Could you check a few things on this model? Use its own coordinates, in mm. Give positions to 0.01 mm unless a question says otherwise; leave off trailing zeros. Loops run counter-clockwise (first coordinate to the right, second up) from the corner with the lowest first, then second, coordinate; pieces in that order, holes last. Notation, with made-up numbers: (-31.75, 21.5) - (2.25, 21.5) arc R10 ccw to (2.25, 40.5) - close; hole circle Ø9 at (4.25, 44). An arc over 180 degrees is marked (long way). Write each question's results on one line, items separated by ' | '. Start each with the question number.
1) I want a section at D-D, the plane y = 2.15. Count the separate pieces of the cut face and the enclosed holes in it, and give its area (3 significant figures).
2) I'm going to push a flat-ended pin straight in: pin 1 (5 mm diameter, centred on x = 12.5, z = 2, fed in from +Y). Where does the tip first touch, or does it pass through?
3) I want a section at C-C, the plane z = -12. Write out the boundary of the cut face in (x, y), and give its area (3 significant figures).
4) If we mould it in two halves opening along X, with no side actions, what happens to faces 1 (the face through (10.464, 1.318, 3.575)), 2 (the face through (0, 1, 17)), 3 (the face through (-17, 1, 0)), 4 (the face through (14.15, 1.32, -13.99))? For each: +X half, -X half, draft (parallel to the pull), parting line (faces both ways), or undercut.
5) I want a section at B-B, the plane x = -5.5. Write out the boundary of the cut face in (y, z).
6) If I drill on probe 1 along X at (y, z) = (1.95, -6); probe 2 along X at (y, z) = (0.6, -1.5); probe 3 along Z at (x, y) = (-8, 2.25), over which ranges is the centre line in solid material (lowest first)? Write a range as [from, to].
7) I want a section at A-A, the plane x = -1. Write out the boundary of the cut face in (y, z), and give its area (3 significant figures).
from build123d import *

# Parameters (mm, degrees)
SKETCH1_W                        = 34
SKETCH1_H                        = 34
BASE_DEPTH                       = 2.6
BASE_FILLET_R                    = 10
INNER_CUT_DEPTH                  = 25.181811347
INNER_LEFT_PROFILE_DEPTH         = 2.6
SKETCH5_R                        = 1.5
RIVET_HOLE_DEPTH                 = 25.181811347
GROOVED_PARTIAL_CIRCLE_CUT_DEPTH = 25.181811347
ILP_F_R                          = 0.5
IC_F_R                           = 1
ILP_F_OF_MIRROR_INNER_FEATURES_R = 0.5
IC_F_OF_MIRROR_INNER_FEATURES_R  = 1


with BuildPart() as part:
    # Sketch1 → BASE (new body)
    with BuildSketch(Plane(origin=(0, 0, 0), x_dir=(1, 0, 0), z_dir=(0, 1, 0))):
        Rectangle(SKETCH1_W, SKETCH1_H)
    extrude(amount=BASE_DEPTH)

    # BASE FILLET
    base_fillet_edges = [part.edges().sort_by_distance(p)[0] for p in [
        (17, 1.3, 17),
        (-17, 1.3, 17),
        (-17, 1.3, -17),
        (17, 1.3, -17),
    ]]
    fillet(base_fillet_edges, radius=BASE_FILLET_R)

    # Sketch3 → INNER CUT (cut, through all)
    with BuildSketch(Plane(origin=(0, 2.6, 0), x_dir=(1, 0, 0), z_dir=(0, 1, 0))):
        with BuildLine():
            Line((-10, -9.5), (10, -9.5))
            ThreePointArc((10, -9.5), (12.828427125, -8.328427125), (14, -5.5))
            Line((14, -5.5), (14, 7))
            ThreePointArc((14, 7), (11.949747468, 11.949747468), (7, 14))
            Line((7, 14), (-7, 14))
            ThreePointArc((-7, 14), (-11.949747468, 11.949747468), (-14, 7))
            Line((-14, 7), (-14, -5.5))
            ThreePointArc((-14, -5.5), (-12.828427125, -8.328427125), (-10, -9.5))
        make_face()
    extrude(amount=-INNER_CUT_DEPTH, mode=Mode.SUBTRACT)

    # Sketch4 → INNER LEFT PROFILE (add)
    with BuildSketch(Plane(origin=(0, 0, 0), x_dir=(1, 0, 0), z_dir=(0, 1, 0))):
        with BuildLine():
            Line((-4, 2.6), (-4, -9.5))
            Line((-4, -9.5), (0, -9.5))
            Line((0, -9.5), (0, 11))
            Line((0, 11), (-7, 11))
            ThreePointArc((-7, 11), (-9.828427125, 9.828427125), (-11, 7))
            Line((-11, 7), (-11, 0.6))
            ThreePointArc((-11, 0.6), (-11.5, -2.9), (-11, -6.4))
            Line((-11, -6.4), (-7, -6.4))
            ThreePointArc((-7, -6.4), (-6.5, -2.9), (-7, 0.6))
            Line((-7, 0.6), (-7, 2.6))
            ThreePointArc((-7, 2.6), (-5.5, 4.1), (-4, 2.6))
        make_face()
    inner_left_profile = extrude(amount=INNER_LEFT_PROFILE_DEPTH)

    # Sketch5 → RIVET HOLE (cut, through all)
    with BuildSketch(Plane(origin=(0, 2.6, 0), x_dir=(1, 0, 0), z_dir=(0, 1, 0))):
        with Locations(Location((-9, -3.9, 0), (0, 0, 270))):
            Circle(SKETCH5_R)
    rivet_hole = extrude(amount=-RIVET_HOLE_DEPTH, mode=Mode.SUBTRACT)

    # Sketch6 → GROOVED PARTIAL CIRCLE CUT (cut, through all)
    with BuildSketch(Plane(origin=(0, 2.6, 0), x_dir=(1, 0, 0), z_dir=(0, 1, 0))):
        with BuildLine():
            Line((-4, -2.95), (-4, -3.95))
            ThreePointArc((-4, -3.95), (-3.7, -3.45), (-4, -2.95))
        make_face()
    grooved_partial_circle_cut = extrude(amount=-GROOVED_PARTIAL_CIRCLE_CUT_DEPTH, mode=Mode.SUBTRACT)

    # ILP F
    ilp_f_edges = [part.edges().sort_by_distance(p)[0] for p in [
        (-11, 1.3, 6.4),
        (-7, 1.3, 6.4),
    ]]
    fillet(ilp_f_edges, radius=ILP_F_R)

    # IC F
    ic_f_edges = [part.edges().sort_by_distance(p)[0] for p in [
        (-4, 1.3, 9.5),
    ]]
    fillet(ic_f_edges, radius=IC_F_R)

    # MIRROR INNER FEATURES: INNER LEFT PROFILE, RIVET HOLE, GROOVED PARTIAL CIRCLE CUT across plane
    add(inner_left_profile.mirror(Plane(origin=(0, 0, 0), x_dir=(0, 0, 1), z_dir=(1, 0, 0))))
    add(rivet_hole.mirror(Plane(origin=(0, 0, 0), x_dir=(0, 0, 1), z_dir=(1, 0, 0))), mode=Mode.SUBTRACT)
    add(grooved_partial_circle_cut.mirror(Plane(origin=(0, 0, 0), x_dir=(0, 0, 1), z_dir=(1, 0, 0))), mode=Mode.SUBTRACT)

    # ILP F of MIRROR INNER FEATURES
    ilp_f_of_mirror_inner_features_edges = [part.edges().sort_by_distance(p)[0] for p in [
        (11, 1.3, 6.4),
        (7, 1.3, 6.4),
    ]]
    fillet(ilp_f_of_mirror_inner_features_edges, radius=ILP_F_OF_MIRROR_INNER_FEATURES_R)

    # IC F of MIRROR INNER FEATURES
    ic_f_of_mirror_inner_features_edges = [part.edges().sort_by_distance(p)[0] for p in [
        (4, 1.3, 9.5),
    ]]
    fillet(ic_f_of_mirror_inner_features_edges, radius=IC_F_OF_MIRROR_INNER_FEATURES_R)


solid = part.part
Answers:
1) separate pieces: 1 | enclosed holes: 3 | area: 775 mm2
2) pin 1: stops at y = 2.6
3) outline: (-15.66, 0) - (-11.9, 0) - (-11.9, 2.6) - (-15.66, 2.6) - close; (11.9, 0) - (15.66, 0) - (15.66, 2.6) - (11.9, 2.6) - close | area: 19.6 mm2
4) face 1: undercut | face 2: draft | face 3: -X half | face 4: +X half
5) outline: (0, -17) - (2.6, -17) - (2.6, -14) - (0, -14) - close; (0, -11) - (2.6, -11) - (2.6, -4.1) - (0, -4.1) - close; (0, 9.5) - (2.6, 9.5) - (2.6, 17) - (0, 17) - close
6) probe 1: x = [-17, -14], [-11, 11], [14, 17] | probe 2: x = [-17, -14], [-11, -7], [-4, 4], [7, 11], [14, 17] | probe 3: z = [-16.95, -13.93], [-10.87, 2.78], [5.02, 6.4], [9.5, 16.95]
7) outline: (0, -17) - (2.6, -17) - (2.6, -14) - (0, -14) - close; (0, -11) - (2.6, -11) - (2.6, 17) - (0, 17) - close | area: 80.6 mm2
